Read the model definition and answer for the solid it produces. Units are mm, in the model's axes. Give positions to 0.01 mm unless a question says otherwise; leave off trailing zeros. Write each loop counter-clockwise with the first axis right and the second up, starting at its lowest first coordinate (ties: lowest second). Pieces come first, ordered by that corner, then holes. Notation, with made-up numbers: (86, -5.75) - (90, -5.75) arc R20 ccw to (90, 31.25) - close; hole circle Ø3 at (-21.75, 28.5). An arc over 180 degrees is marked (long way). Use CSV: the item, a comma, the result in double quotes. Start each with the question number.
from build123d import *

# Parameters (mm, degrees)
SKETCH1_W           = 152.4
SKETCH1_H           = 130
BOSS_EXTRUDE1_DEPTH = 9.5
SKETCH2_R           = 2.5
SKETCH2_R_2         = 3
CUT_EXTRUDE1_DEPTH  = 10
SKETCH3_R           = 6
CUT_EXTRUDE2_DEPTH  = 10
SKETCH4_R           = 2.25
SKETCH4_R_2         = 12.5
CUT_EXTRUDE3_DEPTH  = 10.5
SKETCH5_R           = 3
CUT_EXTRUDE4_DEPTH  = 10.5
SKETCH6_R           = 5
CUT_EXTRUDE5_DEPTH  = 10.5


with BuildPart() as part:
    # Sketch1 → Boss-Extrude1 (new body)
    with BuildSketch(Plane(origin=(0, 0, 0), x_dir=(1, 0, 0), z_dir=(0, 1, 0))):
        Rectangle(SKETCH1_W, SKETCH1_H)
    extrude(amount=BOSS_EXTRUDE1_DEPTH)

    # Sketch2 → Cut-Extrude1 (cut)
    with BuildSketch(Plane(origin=(0, 0, 0), x_dir=(-1, 0, 0), z_dir=(0, -1, 0))):
        with Locations((-4.75, -59.35)):
            Circle(SKETCH2_R)
        with Locations((-51.85, -59.35)):
            Circle(SKETCH2_R_2)
        with Locations((-4.75, -12.25)):
            Circle(SKETCH2_R_2)
        with Locations((-51.85, -12.25)):
            Circle(SKETCH2_R_2)
    extrude(amount=-CUT_EXTRUDE1_DEPTH, mode=Mode.SUBTRACT)

    # Sketch3 → Cut-Extrude2 (cut)
    with BuildSketch(Plane(origin=(0, 9.5, 0), x_dir=(1, 0, 0), z_dir=(0, 1, 0))):
        with Locations((28.3, -35.8)):
            Circle(SKETCH3_R)
    extrude(amount=-CUT_EXTRUDE2_DEPTH, mode=Mode.SUBTRACT)

    # Sketch4 → Cut-Extrude3 (cut, through all)
    with BuildSketch(Plane(origin=(0, 9.5, 0), x_dir=(1, 0, 0), z_dir=(0, 1, 0))):
        with Locations((-26.534128982, -7.921988471)):
            Circle(SKETCH4_R)
        with Locations((13.721874775, 5.705342944)):
            Circle(SKETCH4_R)
        with Locations((0, 47.8)):
            Circle(SKETCH4_R_2)
    extrude(amount=-CUT_EXTRUDE3_DEPTH, mode=Mode.SUBTRACT)

    # Sketch5 → Cut-Extrude4 (cut, through all)
    with BuildSketch(Plane(origin=(0, 9.5, 0), x_dir=(1, 0, 0), z_dir=(0, 1, 0))):
        with Locations((23, 28.65)):
            Circle(SKETCH5_R)
        with Locations((-23, 28.65)):
            Circle(SKETCH5_R)
        with Locations((23, 48.65)):
            Circle(SKETCH5_R)
        with Locations((-23, 48.65)):
            Circle(SKETCH5_R)
    extrude(amount=-CUT_EXTRUDE4_DEPTH, mode=Mode.SUBTRACT)

    # Sketch6 → Cut-Extrude5 (cut, through all)
    with BuildSketch(Plane(origin=(0, 9.5, 0), x_dir=(1, 0, 0), z_dir=(0, 1, 0))):
        with Locations((-66.5, 31.55)):
            Circle(SKETCH6_R)
        with Locations((-66.5, -45.45)):
            Circle(SKETCH6_R)
        with Locations((66.5, -45.45)):
            Circle(SKETCH6_R)
        with Locations((66.5, 31.55)):
            Circle(SKETCH6_R)
        with Locations((-42.5, 13.3)):
            Circle(SKETCH6_R)
        with Locations((42.5, 13.3)):
            Circle(SKETCH6_R)
    extrude(amount=-CUT_EXTRUDE5_DEPTH, mode=Mode.SUBTRACT)


solid = part.part
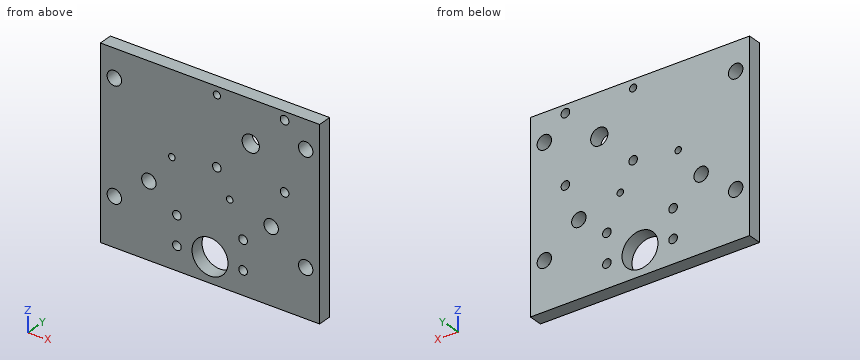
(1) The part is cut by section B-B on x = -66.5. Write down the section's boundary in (y, z).
(2) Consider probe 1 along X at (y, z) = (6, -13.3); probe 2 along Z at (x, y) = (51.85, 6.75); probe 3 along X at (y, z) = (5, -17). Determine where each line is inside the solid, lowest interval first.
(3) The part is cut by section D-D on z = 35.8. Write down the section's boundary in (x, y).
(4) Given P1, Ø7, axis at x = 51.85, z = 59.35, coming from the +Y side, flat-ended and moving along its own axis, determine where the tip first touches the part or whether it passes through.
(5) The part is cut by section A-A on x = 28.3. Write down the section's boundary in (y, z), plus the area to 3 significant figures.
(6) The part is cut by section C-C on z = -13.3. Write down the section's boundary in (x, y), plus the area to 3 significant figures.
Reported:
1,outline,"(0, -65) - (9.5, -65) - (9.5, -36.55) - (0, -36.55) - close; (0, -26.55) - (9.5, -26.55) - (9.5, 40.45) - (0, 40.45) - close; (0, 50.45) - (9.5, 50.45) - (9.5, 65) - (0, 65) - close"
2,probe 1,"-76.2 to -47.5, -37.5 to 37.5, 47.5 to 76.2"
2,probe 2,"-65 to 9.25, 15.25 to 56.35, 62.35 to 65"
2,probe 3,"-76.2 to -45.86, -39.14 to 39.14, 45.86 to 76.2"
3,outline,"(-76.2, 0) - (22.3, 0) - (22.3, 9.5) - (-76.2, 9.5) - close; (34.3, 0) - (76.2, 0) - (76.2, 9.5) - (34.3, 9.5) - close"
4,P1,"y = 9.5"
5,outline,"(0, -65) - (9.5, -65) - (9.5, 29.8) - (0, 29.8) - close; (0, 41.8) - (9.5, 41.8) - (9.5, 65) - (0, 65) - close"
5,area,"1,120 mm²"
6,outline,"(-76.2, 0) - (-47.5, 0) - (-47.5, 9.5) - (-76.2, 9.5) - close; (-37.5, 0) - (37.5, 0) - (37.5, 9.5) - (-37.5, 9.5) - close; (47.5, 0) - (76.2, 0) - (76.2, 9.5) - (47.5, 9.5) - close"
6,area,"1,260 mm²"
